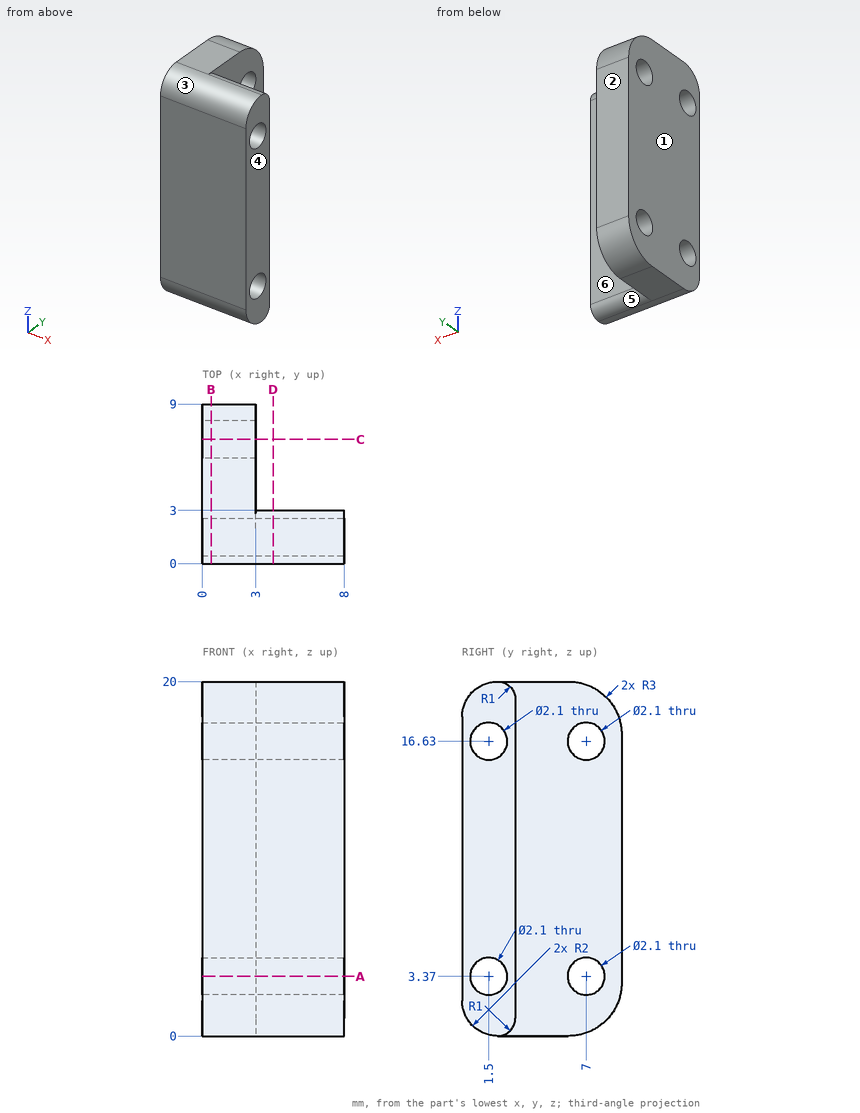
The drawing under review shows one solid part. Ordinate dimensions are in mm from its lowest x, y, z. A direction names the side the tool comes from. Round coordinates to 2 decimals unless told otherwise and drop trailing zeros. Loops run counter-clockwise (first coordinate to the right, second up) from the corner with the lowest first, then second, coordinate; pieces in that order, holes last. Notation, with made-up numbers: (-22.5, -33.5) - (2.5, -33.5) arc R19 ccw to (2.5, -25.5) - close; hole circle Ø7 at (86.25, 79.5). An arc over 180 degrees is marked (long way). Put each result on its own line as item: value. Start each with the question number.
1. For the marked faces 4, 5 and 6, list the 3-axis set-ups (+Z, -Z, +X, -X, +Y, -Y) from which the entire face can be reached by the end or side of a thin tool; tool diameter is ignored.
2. Consider section C-C on y = 7. State the section outline as (x, z) points, plus the area to 3 significant figures.
3. Insertion check: P1, Ø1.9, axis at y = 1.5, z = 3.37, coming from the +X side; P2, Ø3.5, axis at y = 6.5, z = 10.5, coming from the +X side; P3, Ø1.5, axis at x = 3.5, y = 7.5, coming from the -Z side; P4, Ø2, axis at x = 6.5, z = 11, coming from the +Y side. Each pin has a flat end and moves straight along its axis. Give the tip position at first contact, or say it passes through.
4. Consider section D-D on x = 4. State how many separate pieces and enclosed holes the cut face has, plus the area to 3 significant figures.
5. For probe 1 along Y at (x, z) = (0.6, 3.37); probe 2 along Y at (x, z) = (3.5, 16.63); probe 3 along Y at (x, z) = (7.25, 14), list the stretches that pass through material, from the lowest coordinate up. Write a range as [from, to].
6. Mouldability with a two-part tool opening along Y and no side actions: class the marked faces 1, 2 and 3 as +Y half, -Y half, draft (parallel to the pull), parting line (faces both ways), or undercut.
7. Consider section A-A on z = 3.37. State the section outline as (x, y) points, plus the area to 3 significant figures.
8. Consider section B-B on x = 0.5. State the section outline as (y, z) points.
Result sheet:
1. face 4: +Z, -Z, +X, +Y, -Y
1. face 5: -Z, +X, +Y
1. face 6: +Z, -Z, +X, +Y
2. outline: (0, 0.17) - (3, 0.17) - (3, 2.32) - (0, 2.32) - close; (0, 4.42) - (3, 4.42) - (3, 15.58) - (0, 15.58) - close; (0, 17.68) - (3, 17.68) - (3, 19.83) - (0, 19.83) - close
2. area: 46.4 mm^2
3. P1: through
3. P2: x = 3
3. P3: z = 0.15
3. P4: y = 3
4. separate pieces: 1
4. enclosed holes: 2
4. area: 50.9 mm^2
5. probe 1: [0, 0.45], [2.55, 5.95], [8.05, 9]
5. probe 2: [0, 0.45], [2.55, 3]
5. probe 3: [0, 3]
6. face 1: draft
6. face 2: +Y half
6. face 3: -Y half
7. outline: (0, 0) - (8, 0) - (8, 0.45) - (0, 0.45) - close; (0, 2.55) - (8, 2.55) - (8, 3) - (3, 3) - (3, 5.95) - (0, 5.95) - close; (0, 8.05) - (3, 8.05) - (3, 9) - (0, 9) - close
7. area: 18.9 mm^2
8. outline: (0, 2) arc R2 ccw to (2, 0) - (6, 0) arc R3 ccw to (9, 3) - (9, 17) arc R3 ccw to (6, 20) - (2, 20) arc R2 ccw to (0, 18) - close; hole circle Ø2.1 at (1.5, 3.37); hole circle Ø2.1 at (1.5, 16.63); hole circle Ø2.1 at (7, 3.37); hole circle Ø2.1 at (7, 16.63)
